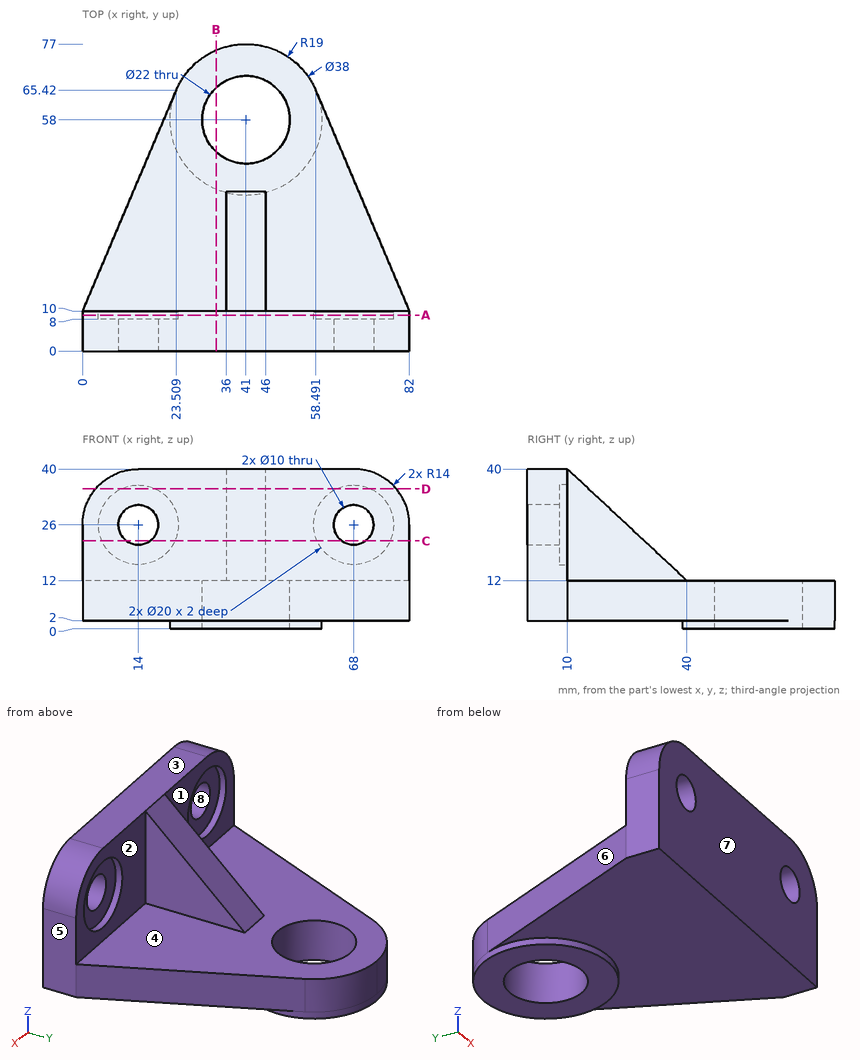
Input: dimensioned drawing with shaded views. Units: mm. Origin: part minimum x, y, z. A direction names the side the tool comes from. Give positions to 0.01 mm unless a question says otherwise; leave off trailing zeros. Loops run counter-clockwise (first coordinate to the right, second up) from the corner with the lowest first, then second, coordinate; pieces in that order, holes last. Notation, with made-up numbers: (-40, 62) -> (-22, 62) arc R25 ccw to (-22, 79) -> close; hole circle Ø2 at (3.25, 61.5). An arc over 180 degrees is marked (long way). Use a Markdown table: item, result.
Q1. Access query for the marked faces 1, 2, 3, 4 and 5. Directions: +Z, -Z, +X, -X, +Y, -Y. A direction counts if a zero-diameter tool reaches every point of the face in a straight line with its end or side. Return the directions, or none.
Entries:
| item | result |
|---|---|
| face 1 | +Z, -X, +Y |
| face 2 | +Z, +X, +Y |
| face 3 | +Z, +X, -X, +Y, -Y |
| face 4 | +Z, +Y |
| face 5 | +Z, -Z, +X, +Y, -Y |
Q2. Pull-direction query (X, two-part tool) for the marked faces 6, 7 and 8; classes: pulls with the +X half, pulls with the -X half, needs draft (parallel to the pull), parting line crosses it, or undercut.
Entries:
| item | result |
|---|---|
| face 6 | pulls with the -X half |
| face 7 | needs draft |
| face 8 | undercut |
Q3. Section query D-D, the plane z = 35. Return the cut outline in (x, y), plus the area to 3 significant figures.
Entries:
| item | result |
|---|---|
| outline | (3.28, 0) -> (78.72, 0) -> (78.72, 10) -> (72.36, 10) -> (72.36, 8) -> (63.64, 8) -> (63.64, 10) -> (46, 10) -> (46, 15.36) -> (36, 15.36) -> (36, 10) -> (18.36, 10) -> (18.36, 8) -> (9.64, 8) -> (9.64, 10) -> (3.28, 10) -> close |
| area | 773 mm² |
Q4. Section query B-B, the plane x = 33.5. Return the cut outline in (y, z).
Entries:
| item | result |
|---|---|
| outline | (0, 2) -> (40.54, 2) -> (40.54, 0) -> (49.95, 0) -> (49.95, 12) -> (10, 12) -> (10, 40) -> (0, 40) -> close; (66.05, 0) -> (75.46, 0) -> (75.46, 12) -> (66.05, 12) -> close |
Q5. Section query C-C, the plane z = 22. Return the cut outline in (x, y) (1 decimal).
Entries:
| item | result |
|---|---|
| outline | (0, 0) -> (11, 0) -> (11, 8) -> (4.8, 8) -> (4.8, 10) -> (0, 10) -> close; (17, 0) -> (65, 0) -> (65, 8) -> (58.8, 8) -> (58.8, 10) -> (46, 10) -> (46, 29.3) -> (36, 29.3) -> (36, 10) -> (23.2, 10) -> (23.2, 8) -> (17, 8) -> close; (71, 0) -> (82, 0) -> (82, 10) -> (77.2, 10) -> (77.2, 8) -> (71, 8) -> close |
Q6. Ray query, probe 1 along X at (y, z) = (6, 26); probe 2 along Y at (x, z) = (41, 5.75); probe 3 along Z at (x, y) = (14, 5). Return the intervals inside material, ascending. Write a range as from..to.
Entries:
| item | result |
|---|---|
| probe 1 | x = 0..9, 19..63, 73..82 |
| probe 2 | y = 0..47, 69..77 |
| probe 3 | z = 2..21, 31..40 |
Q7. Section query A-A, the plane y = 9. Return the cut outline in (x, z).
Entries:
| item | result |
|---|---|
| outline | (0, 2) -> (82, 2) -> (82, 26) arc R14 ccw to (68, 40) -> (14, 40) arc R14 ccw to (0, 26) -> close; hole circle Ø20 at (14, 26); hole circle Ø20 at (68, 26) |
Q8. First-contact query: P1, Ø16, axis at x = 14, z = 26, coming from the +Y side; P2, Ø8.5, axis at y = 28.5, z = 27.5, coming from the +X side; P3, Ø8, axis at x = 15, y = 51.5, coming from the -Z side. Flat tips, straight axial feed; report the tip coordinate or a pass-through.
Entries:
| item | result |
|---|---|
| P1 | stops at y = 8 |
| P2 | stops at x = 46 |
| P3 | stops at z = 2 |
